Source: three-view drawing plus pictorial views. Frame: mm from the lowest corner of the part. A direction names the side the tool comes from. Round coordinates to 2 decimals unless told otherwise and drop trailing zeros. Order: outer loops, then holes, each group sorted by start corner. A loop starts at its lowest first (then second) coordinate and runs counter-clockwise, first axis right, second up. Notation, with made-up numbers: M 6,-5.5 L 61,-5.5 A21 ccw 61,23.5 Z; hole C 87,33 d3. An arc over 180 degrees is marked long. Return JSON: item names as keys, results as strings. Group by question number.
Q1. Ray query, probe 1 along Y at (x, z) = (15.5, 16.7); probe 2 along Y at (x, z) = (15.5, 5.5); probe 3 along X at (y, z) = (75.5, 7.75). Return the intervals inside material, ascending.
Q2. Cut plane D-D on y = 7. Output: boundary loops of the cut face in (x, z), and give its area (4 significant figures).
Q3. Cut plane B-B on x = 15.5. Output: boundary loops of the cut face in (y, z).
Q4. Mould query, pull axis X, two halves, no side actions, for the marked faces 1, 2 and 3. Classes: released by +X, released by -X, zero draft, split by the parting line, or undercut.
Q5. Contact query for flat-ended pins moving along their axis: pin 1 (7.5 mm diameter, centred on x = 15.5, y = 15, fed in from +Z); pin 2 (4 mm diameter, centred on y = 58, z = 10, fed in from -X); pin 3 (2 mm diameter, centred on x = 6.5, y = 26.5, fed in from -Z); pin 4 (6 mm diameter, centred on x = 15.5, y = 65, fed in from -Z). Output: stop coordinate, or through.
Q6. Access query for the marked faces 4, 5 and 6. Directions: +Z, -Z, +X, -X, +Y, -Y. A direction counts if a zero-diameter tool reaches every point of the face in a straight line with its end or side. Return the directions, or none.
Q7. Cut plane C-C on z = 9.75. Output: boundary loops of the cut face in (x, y), and give its area (3 significant figures).
Q8. Cut plane A-A on y = 15. Output: boundary loops of the cut face in (x, z), and give its area (4 significant figures).
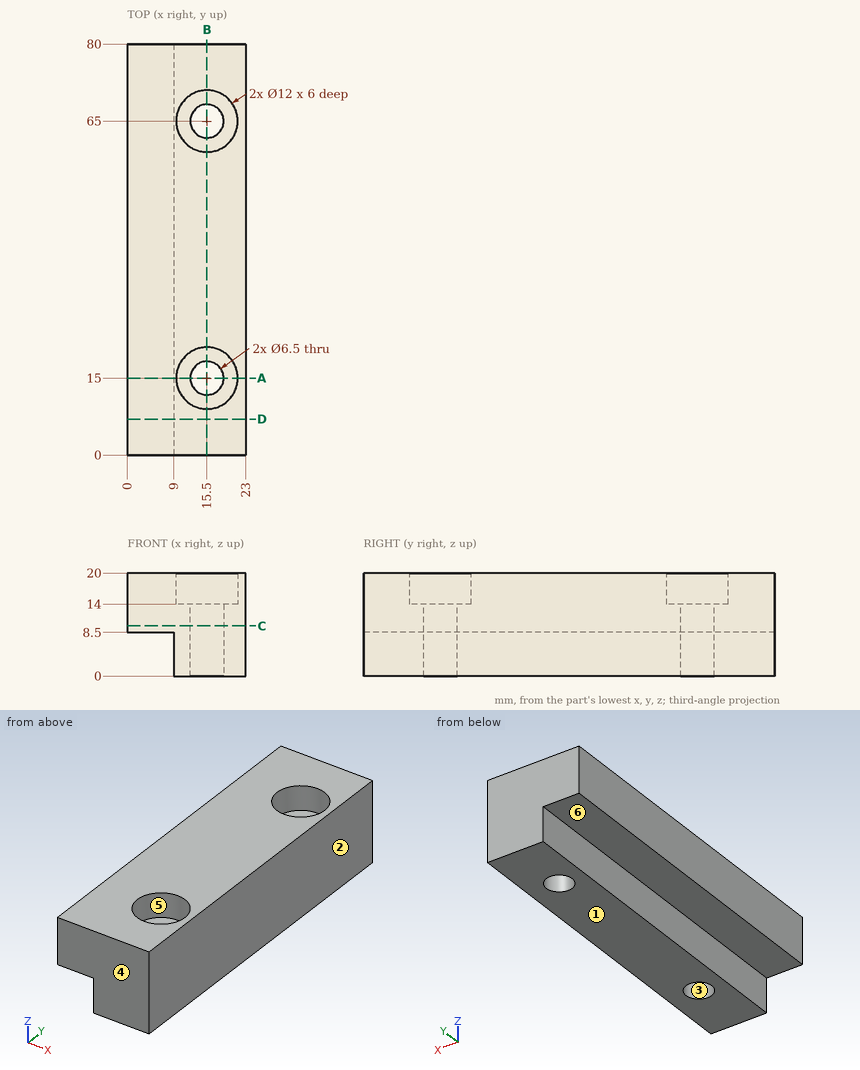
Result sheet:
{
 "1": {"probe 1": "y = 0 to 9, 21 to 59, 71 to 80", "probe 2": "y = 0 to 11.75, 18.25 to 61.75, 68.25 to 80", "probe 3": "x = 9 to 23"},
 "2": {"outline": "M 0,8.5 L 9,8.5 L 9,0 L 23,0 L 23,20 L 0,20 Z", "area": "383.5 mm²"},
 "3": {"outline": "M 0,0 L 11.75,0 L 11.75,14 L 9,14 L 9,20 L 0,20 Z; M 18.25,0 L 61.75,0 L 61.75,14 L 59,14 L 59,20 L 21,20 L 21,14 L 18.25,14 Z; M 68.25,0 L 80,0 L 80,20 L 71,20 L 71,14 L 68.25,14 Z"},
 "4": {"face 1": "zero draft", "face 2": "released by +X", "face 3": "undercut"},
 "5": {"pin 1": "stops at z = 14", "pin 2": "stops at x = 0", "pin 3": "stops at z = 8.5", "pin 4": "passes through"},
 "6": {"face 4": "+Z, -Z, +X, -X, -Y", "face 5": "+Z", "face 6": "-Z, -X, +Y, -Y"},
 "7": {"outline": "M 0,0 L 23,0 L 23,80 L 0,80 Z; hole C 15.5,15 d6.5; hole C 15.5,65 d6.5", "area": "1,770 mm²"},
 "8": {"outline": "M 0,8.5 L 9,8.5 L 9,0 L 12.25,0 L 12.25,14 L 9.5,14 L 9.5,20 L 0,20 Z; M 18.75,0 L 23,0 L 23,20 L 21.5,20 L 21.5,14 L 18.75,14 Z", "area": "220.5 mm²"}
}
